from build123d import *


with BuildPart() as part:
    # Esquisse1 → Révolution1 (revolve)
    with BuildSketch(Plane(origin=(0, 0, 0), x_dir=(0, 0, -1), z_dir=(1, 0, 0)), mode=Mode.PRIVATE) as r_volution1_sk:
        Polygon((-2.6, 19), (-2.6, 15.5), (-3.6, 15.5), (-3.6, 13.5), (-2.55, 13.5), (-2.55, 9), (-7.5, 9), (-13.75, 6), (-7.5, 3.2), (-15, 0), (-15, 0.9), (-9.611144406, 3.2), (-15.75, 5.2), (-15.75, 6.8), (-9, 9.7), (-9, 19), align=None)
    revolve(r_volution1_sk.sketch.rotate(Axis((0, 0, 0), (0, 1, 0)), 180), axis=Axis((0, 0, 0), (0, 1, 0)))


solid = part.part
Read the model definition and answer for the solid it produces. Units are mm, in the model's axes. A direction names the side the tool comes from. Give positions to 0.01 mm unless a question says otherwise; leave off trailing zeros. Write each loop counter-clockwise with the first axis right and the second up, starting at its lowest first coordinate (ties: lowest second). Pieces come first, ordered by that corner, then holes. Notation, with made-up numbers: M -12.75,25.25 L 26.25,25.25 A35 ccw 26.25,62.25 Z; hole C 44,-17.5 d5. An arc over 180 degrees is marked long. One line per item, written item: value. Start each with the question number.
(1) Find section C-C (y = 16). Determine the outline of the cut face in (x, z).
(2) Find section D-D (z = -10). Give the number of separate pieces and of enclosed holes in the cut face, plus the area to 3 significant figures.
(3) Find the intervals of material crossed by line 1 (Y direction, x = 10, z = 6.5); line 2 (Y direction, x = -5, z = -11); line 3 (X direction, y = 11.25, z = 0), in increasing order.
(4) Determine the mould class of faces 5 (the flat face through (2, 19, -2)), 6 (the conical face through (7.618, 3.336, 1.692)), 7 (the conical face through (-2.37, 8.81, -7.53)), 8 (the cylindrical face through (-0.77, 11.22, -2.43)) for opening direction Y: pulls with the +Y half, pulls with the -Y half, needs draft (parallel to the pull), parting line crosses it, or undercut.
(5) Flat-ended cylindrical pins translate along their axes: pin 1 Ø6 at (y, z) = (5.5, 4) entering from +X; pin 2 Ø4 at (x, z) = (3, -9) entering from -Y; pin 3 Ø16.5 at (x, z) = (1, 0.5) entering from -Y; pin 4 Ø4 at (x, z) = (0, 0) entering from -Y. Find the tip coordinate at first contact, or state that the pin passes through.
(6) A tool of negligible diameter and unlimited length cuts with its end or side. For faces 1 (the cylindrical face through (-6.083, 14.415, 6.633)), 2 (the cylindrical face through (-1.081, 14.486, -3.434)), 3 (the cylindrical face through (-15.616, 6.011, 2.05)), 4 (the flat face through (0, 9, 3)), from which of +Z, -Z, +X, -X, +Y, -Y can it reach the whole face along a straight path? Write none if from no direction.
Results below:
1. outline: C 0,0 d18; hole C 0,0 d5.2
2. separate pieces: 2
2. enclosed holes: 1
2. area: 83.9 mm^2
3. line 1: y = 1.31 to 2.21, 3.95 to 5.18, 6.88 to 8.44
3. line 2: y = 1.24 to 2.14, 4.01 to 5.25, 6.8 to 8.38
3. line 3: x = -9 to -2.55, 2.55 to 9
4. face 5: pulls with the +Y half
4. face 6: undercut
4. face 7: undercut
4. face 8: needs draft
5. pin 1: stops at x = 15.72
5. pin 2: stops at y = 1.5
5. pin 3: stops at y = 2.4
5. pin 4: passes through
6. face 1: +Y
6. face 2: none
6. face 3: +Y, -Y
6. face 4: -Y
